```python
from build123d import *

# Parameters (mm, degrees)
CROQUIS5_R            = 1.5
CORTAR_EXTRUIR1_DEPTH = 19


with BuildPart() as part:
    # Croquis1 → Recubrir1 section 0
    with BuildSketch(Plane(origin=(0, 0, 0), x_dir=(1, 0, 0), z_dir=(0, 1, 0))):
        with BuildLine():
            Line((-6.045907789, 0), (-4.891242148, -3.553695435))
            Line((-4.891242148, -3.553695435), (-1.868288253, -5.75))
            Line((-1.868288253, -5.75), (1.868288253, -5.75))
            Line((1.868288253, -5.75), (4.891242148, -3.553695435))
            Line((4.891242148, -3.553695435), (6.045907789, 0))
            Line((6.045907789, 0), (4.891242148, 3.553695435))
            Line((4.891242148, 3.553695435), (1.868288253, 5.75))
            Line((1.868288253, 5.75), (-1.868288253, 5.75))
            Line((-1.868288253, 5.75), (-4.891242148, 3.553695435))
            Line((-4.891242148, 3.553695435), (-6.045907789, 0))
        make_face()
    # Croquis2 → Recubrir1 section 1
    with BuildSketch(Plane(origin=(0, 17.3, 0), x_dir=(1, 0, 0), z_dir=(0, 1, 0))):
        with BuildLine():
            Line((-8.936753451, 0.109878116), (-7.294570153, -5.163998619))
            Line((-7.294570153, -5.163998619), (-2.866108989, -8.465403399))
            Line((-2.866108989, -8.465403399), (2.657108393, -8.53331181))
            Line((2.657108393, -8.53331181), (7.16540068, -5.341785145))
            Line((7.16540068, -5.341785145), (8.936753451, -0.109878116))
            Line((8.936753451, -0.109878116), (7.294570153, 5.163998619))
            Line((7.294570153, 5.163998619), (2.866108989, 8.465403399))
            Line((2.866108989, 8.465403399), (-2.657108393, 8.53331181))
            Line((-2.657108393, 8.53331181), (-7.16540068, 5.341785145))
            Line((-7.16540068, 5.341785145), (-8.936753451, 0.109878116))
        make_face()
    loft()

    # Croquis4 → Recubrir2 section 0
    with BuildSketch(Plane(origin=(0, 19.3, 0), x_dir=(1, 0, 0), z_dir=(0, 1, 0))):
        with BuildLine():
            Line((-0.525731112, 0), (-0.425325404, -0.309016994))
            Line((-0.425325404, -0.309016994), (-0.162459848, -0.5))
            Line((-0.162459848, -0.5), (0.162459848, -0.5))
            Line((0.162459848, -0.5), (0.425325404, -0.309016994))
            Line((0.425325404, -0.309016994), (0.525731112, 0))
            Line((0.525731112, 0), (0.425325404, 0.309016994))
            Line((0.425325404, 0.309016994), (0.162459848, 0.5))
            Line((0.162459848, 0.5), (-0.162459848, 0.5))
            Line((-0.162459848, 0.5), (-0.425325404, 0.309016994))
            Line((-0.425325404, 0.309016994), (-0.525731112, 0))
        make_face()
    # Croquis2_3 → Recubrir2 section 1
    with BuildSketch(Plane(origin=(0, 17.3, 0), x_dir=(1, 0, 0), z_dir=(0, 1, 0))):
        with BuildLine():
            Line((-8.936753451, 0.109878116), (-7.294570153, -5.163998619))
            Line((-7.294570153, -5.163998619), (-2.866108989, -8.465403399))
            Line((-2.866108989, -8.465403399), (2.657108393, -8.53331181))
            Line((2.657108393, -8.53331181), (7.16540068, -5.341785145))
            Line((7.16540068, -5.341785145), (8.936753451, -0.109878116))
            Line((8.936753451, -0.109878116), (7.294570153, 5.163998619))
            Line((7.294570153, 5.163998619), (2.866108989, 8.465403399))
            Line((2.866108989, 8.465403399), (-2.657108393, 8.53331181))
            Line((-2.657108393, 8.53331181), (-7.16540068, 5.341785145))
            Line((-7.16540068, 5.341785145), (-8.936753451, 0.109878116))
        make_face()
    loft()

    # Croquis5 → Cortar-Extruir1 (cut)
    with BuildSketch(Plane.XZ):
        with Locations(Location((0, 0, 0), (0, 0, 270))):
            Circle(CROQUIS5_R)
    extrude(amount=-CORTAR_EXTRUIR1_DEPTH, mode=Mode.SUBTRACT)


solid = part.part
```
For this review, take the finished solid that the model builds, in its own axes (mm). Give positions to 0.01 mm unless a question says otherwise; leave off trailing zeros. Answer as a JSON object with one key per item and string values. Group by question number.
Item 1: For pin 1 Ø1.5 at (x, y) = (-1.5, 11.5) entering from +Z; pin 2 Ø10 at (x, y) = (-6.5, 13.5) entering from +Z; pin 3 Ø4 at (x, z) = (4, 5.5) entering from +Y; pin 4 Ø5 at (x, z) = (0, 0) entering from -Y, all flat-tipped, find the tip position at first contact; note any pin that passes through.
Item 2: Draft analysis for pull direction X (two halves, no side actions). For faces 1 (the flat face through (1.3, 0, -1.2)), 2 (the cylindrical face through (0.45, 9.37, -1.43)), 3 (the flat face through (0, 19, 0)), state which applies: +X half, -X half, draft (parallel to the pull), parting line (faces both ways), or undercut.
Item 3: For probe 1 along X at (y, z) = (15.25, 0); probe 2 along X at (y, z) = (15, 0); probe 3 along Z at (x, y) = (-0.5, 11.25), list the stretches that pass through material, from the lowest coordinate up. Write a range as [from, to].
Check result:
{
 "1": {"pin 1": "stops at z = 7.68", "pin 2": "stops at z = 8.4", "pin 3": "stops at y = 18.22", "pin 4": "stops at y = 0"},
 "2": {"face 1": "draft", "face 2": "undercut", "face 3": "undercut"},
 "3": {"probe 1": "x = [-8.56, -1.5], [1.5, 8.56]", "probe 2": "x = [-8.52, -1.5], [1.5, 8.52]", "probe 3": "z = [-7.54, -1.41], [1.41, 7.53]"}
}
